Design review of the part built by this model. Coordinates are the model's own, in mm. A direction names the side the tool comes from. Coordinates: 2 decimals unless noted, no trailing zeros. Loops run counter-clockwise (first coordinate to the right, second up) from the corner with the lowest first, then second, coordinate; pieces in that order, holes last.
from build123d import *
from build123d.topology import SkipClean

# Parameters (mm, degrees)
SKETCH1_W           = 60
SKETCH1_H           = 60
BOSS_EXTRUDE1_DEPTH = 3
SKETCH4_W           = 8
SKETCH4_H           = 12
SKETCH4_W_2         = 12
SKETCH4_H_2         = 8
BOSS_EXTRUDE3_DEPTH = 41
SKETCH5_R           = 2
CUT_EXTRUDE2_DEPTH  = 6
SKETCH8_R           = 7.5
CUT_EXTRUDE4_DEPTH  = 6
CUT_EXTRUDE5_DEPTH  = 6
CUT_EXTRUDE6_DEPTH  = 6
SKETCH11_W          = 23.25
SKETCH11_H          = 3
CUT_EXTRUDE7_DEPTH  = 6
SKETCH12_R          = 3
CUT_EXTRUDE8_DEPTH  = 2
SKETCH13_R          = 1.75
CUT_EXTRUDE9_DEPTH  = 1
CHAMFER1_SIZE       = 2
CHAMFER2_SIZE       = 2
CHAMFER3_SIZE       = 2
CUT_EXTRUDE10_DEPTH = 10
FILLET1_R           = 10
CUT_EXTRUDE11_DEPTH = 59.999486357


with BuildPart() as part:
    # Sketch1 → Boss-Extrude1 (new body)
    with BuildSketch(Plane(origin=(0, 0, 0), x_dir=(1, 0, 0), z_dir=(0, 1, 0))):
        Rectangle(SKETCH1_W, SKETCH1_H)
    extrude(amount=BOSS_EXTRUDE1_DEPTH)

    # Sketch4 → Boss-Extrude3 (add)
    with BuildSketch(Plane.XZ):
        with Locations((-26, 0)):
            Rectangle(SKETCH4_W, SKETCH4_H)
        with Locations((0, -26)):
            Rectangle(SKETCH4_W_2, SKETCH4_H_2)
        with Locations((26, 0)):
            Rectangle(SKETCH4_W, SKETCH4_H)
    extrude(amount=BOSS_EXTRUDE3_DEPTH)

    # Sketch5 → Cut-Extrude2 (cut)
    with BuildSketch(Plane.XZ.offset(41)):
        with Locations(Location((0, -26.5, 0), (0, 0, 270))):
            Circle(SKETCH5_R)
        with Locations(Location((-26.5, 0, 0), (0, 0, 270))):
            Circle(SKETCH5_R)
        with Locations(Location((26.5, 0, 0), (0, 0, 270))):
            Circle(SKETCH5_R)
    extrude(amount=-CUT_EXTRUDE2_DEPTH, mode=Mode.SUBTRACT)

    # Sketch8 → Cut-Extrude4 (cut)
    with BuildSketch(Plane(origin=(0, 3, 0), x_dir=(1, 0, 0), z_dir=(0, 1, 0))):
        with Locations(Location((0, 0, 0), (0, 0, 270))):
            Circle(SKETCH8_R)
    extrude(amount=-CUT_EXTRUDE4_DEPTH, mode=Mode.SUBTRACT)

    # Sketch7 → Cut-Extrude5 (cut)
    with BuildSketch(Plane.XZ):
        Polygon((-30, -6), (-6, -30), (-30, -30), align=None)
        Polygon((30, -6), (6, -30), (30, -30), align=None)
    extrude(amount=-CUT_EXTRUDE5_DEPTH, mode=Mode.SUBTRACT)

    # Sketch10 → Cut-Extrude6 (cut)
    with BuildSketch(Plane.XZ):
        Polygon((-9, 30), (-30, 6), (-30, 30), align=None)
        Polygon((9, 30), (30, 6), (30, 30), align=None)
    extrude(amount=-CUT_EXTRUDE6_DEPTH, mode=Mode.SUBTRACT)

    # Sketch11 → Cut-Extrude7 (cut)
    with BuildSketch(Plane.XZ):
        with Locations((0, 28.5)):
            Rectangle(SKETCH11_W, SKETCH11_H)
    extrude(amount=-CUT_EXTRUDE7_DEPTH, mode=Mode.SUBTRACT)

    # Sketch12 → Cut-Extrude8 (cut)
    with BuildSketch(Plane.XZ):
        with Locations(Location((-8, 8, 0), (0, 0, 270))):
            Circle(SKETCH12_R)
        with Locations(Location((8, 8, 0), (0, 0, 270))):
            Circle(SKETCH12_R)
        with Locations(Location((8, -8, 0), (0, 0, 270))):
            Circle(SKETCH12_R)
        with Locations(Location((-8, -8, 0), (0, 0, 270))):
            Circle(SKETCH12_R)
    extrude(amount=-CUT_EXTRUDE8_DEPTH, mode=Mode.SUBTRACT)

    # Sketch13 → Cut-Extrude9 (cut)
    with BuildSketch(Plane(origin=(0, 3, 0), x_dir=(1, 0, 0), z_dir=(0, 1, 0))):
        with Locations(Location((-8, 8, 0), (0, 0, 270))):
            Circle(SKETCH13_R)
        with Locations(Location((8, 8, 0), (0, 0, 270))):
            Circle(SKETCH13_R)
        with Locations(Location((8, -8, 0), (0, 0, 270))):
            Circle(SKETCH13_R)
        with Locations(Location((-8, -8, 0), (0, 0, 270))):
            Circle(SKETCH13_R)
    extrude(amount=-CUT_EXTRUDE9_DEPTH, mode=Mode.SUBTRACT)

    # Chamfer1
    chamfer1_edges = [part.edges().sort_by_distance(p)[0] for p in [
        (30, 3, 0),
        (0, 3, -30),
        (-30, 3, 0),
    ]]
    chamfer(chamfer1_edges, length=CHAMFER1_SIZE)

    # Chamfer2
    chamfer2_edges = [part.edges().sort_by_distance(p)[0] for p in [
        (0, 3, 27),
    ]]
    chamfer(chamfer2_edges, length=CHAMFER2_SIZE)

    # Chamfer3
    chamfer3_edges = [part.edges().sort_by_distance(p)[0] for p in [
        (6, -20.5, -30),
        (-6, -20.5, -30),
        (-30, -20.5, -6),
        (-30, -20.5, 6),
        (30, -20.5, 6),
        (30, -20.5, -6),
    ]]
    chamfer(chamfer3_edges, length=CHAMFER3_SIZE)

    # Sketch14 → Cut-Extrude10 (cut)
    with BuildSketch(Plane.XZ):
        Polygon((-30, -4), (-4, -30), (-6, -30), (-30, -6), align=None)
        Polygon((4, -30), (30, -4), (30, -6), (6, -30), align=None)
    extrude(amount=-CUT_EXTRUDE10_DEPTH, mode=Mode.SUBTRACT)

    # Fillet1
    # the kernel refuses this fillet: 10 mm, written as the material it takes off along each edge
    with BuildSketch(Plane(origin=(-4, 11.355339059, -30), x_dir=(1, 0, 0), z_dir=(0, -1, 0)), Plane(origin=(4, -51.355339059, -30), x_dir=(-1, 0, 0), z_dir=(0, 1, 0)), Plane(origin=(30, 11.355339059, -4), x_dir=(0, 0, 1), z_dir=(0, -1, 0))) as fillet1_piece_1:
        with BuildLine():
            CenterArc((FILLET1_R * 0.414213562373, FILLET1_R), FILLET1_R, 225, 45)
            Line((-FILLET1_R * 0.292893218813, FILLET1_R * 0.292893218813), (0, 0))
            Line((0, 0), (FILLET1_R * 0.414213562373, 0))
        make_face()
    extrude(amount=62.710678119, mode=Mode.SUBTRACT)
    with BuildSketch(Plane(origin=(-30, 0, 4), x_dir=(0, 0, -1), z_dir=(0, -1, 0))) as fillet1_piece_2:
        with BuildLine():
            CenterArc((4, 10), FILLET1_R, 233.130102354, 36.869897646)
            Line((-2, 2), (0, 0))
            Line((0, 0), (4, 0))
        make_face()
    extrude(amount=51, mode=Mode.SUBTRACT)
    with BuildSketch(Plane(origin=(-30, 11.355339059, -4), x_dir=(0, 0, 1), z_dir=(0, -1, 0))) as fillet1_piece_3:
        with BuildLine():
            CenterArc((FILLET1_R * 0.414213562373, -FILLET1_R), FILLET1_R, 90, 45)
            Line((-FILLET1_R * 0.292893218813, -FILLET1_R * 0.292893218813), (0, 0))
            Line((0, 0), (FILLET1_R * 0.414213562373, 0))
        make_face()
    extrude(amount=62.710678119, mode=Mode.SUBTRACT)
    with BuildSketch(Plane(origin=(30, 0, 4), x_dir=(0, 0, -1), z_dir=(0, -1, 0))) as fillet1_piece_4:
        with BuildLine():
            CenterArc((4, -10), FILLET1_R, 90, 36.869897646)
            Line((-2, -2), (0, 0))
            Line((0, 0), (4, 0))
        make_face()
    extrude(amount=51, mode=Mode.SUBTRACT)

    # Sketch16 → Cut-Extrude11 (cut, through all)
    with SkipClean():  # the faces are left unmerged after this step: merging them gives an invalid solid
        with BuildSketch(Plane.XZ):
            with BuildLine():
                Line((-28, 6), (-9.625, 27))
                Line((-9.625, 27), (-11.625, 27))
                Line((-11.625, 27), (-30, 6))
                Line((-30, 6), (-30, 0.142135624))
                ThreePointArc((-30, 0.142135624), (-29.999936866, 0.106601493), (-29.999747465, 0.071067812))
                ThreePointArc((-29.999747465, 0.071067812), (-29.475536208, 3.195968331), (-28, 6))
            make_face()
            with BuildLine():
                Line((28, 6), (9.625, 27))
                Line((9.625, 27), (11.625, 27))
                Line((11.625, 27), (30, 6))
                Line((30, 6), (30, 0.142135624))
                ThreePointArc((30, 0.142135624), (29.999936866, 0.106601493), (29.999747465, 0.071067812))
                ThreePointArc((29.999747465, 0.071067812), (29.475536208, 3.195968331), (28, 6))
            make_face()
        extrude(amount=-CUT_EXTRUDE11_DEPTH, mode=Mode.SUBTRACT)


solid = part.part
Q1. Machinability: for faces 4 (the flat face through (-6, -20, -25)), 5 (the cylindrical face through (24.548, -38.042, 0.434)), 6 (the flat face through (22, -20, 0)), which of the approach directions +Z, -Z, +X, -X, +Y, -Y give a long, thin tool a straight path to every point of the face, cutting with its end or side? Answer none if there is none.
Q2. For line 1 (X direction, y = 2.6, z = -8); line 2 (X direction, y = 0.5, z = -8); line 3 (Y direction, x = -21, z = 13), list the stretches that pass through material, from the lowest coordinate up.
Q3. Take a section at A-A, the plane y = -37.5. Write out the cut boundary in (x, z).
Q4. Take a section at C-C, the plane z = 4. Write out the cut boundary in (x, y).
Q5. Take a section at D-D, the plane x = 25.5. Write out the cut boundary in (y, z), then the cut area to 3 significant figures.
Q6. Clearance check with flat-ended pins moving along their axes: pin 1 Ø3 at (y, z) = (-19.5, -23.5) entering from -X; pin 2 Ø5 at (x, z) = (8.5, -8.5) entering from -Y; pin 3 Ø5 at (x, y) = (-3, -3.5) entering from -Z. State where each tip first meets the part, or that it passes through.
Q7. The part is to be moulded in two halves that separate along Z. For faces 1 (the flat face through (29, 2, 0)), 2 (the cylindrical face through (2.999, -19.308, -29.494)), 3 (the flat face through (-8, 2, 6)), say which applies: pulls with the +Z half, pulls with the -Z half, needs draft (parallel to the pull), parting line crosses it, or undercut.
Q8. Take a section at B-B, the plane x = 4. Write out the cut boundary in (y, z), then the cut area to 3 significant figures.
Entries:
1. face 4: +Z, -Z, -X, -Y
1. face 5: -Y
1. face 6: +Z, -Z, -Y
2. line 1: x = -26 to -9.75, -6.25 to 6.25, 9.75 to 26
2. line 2: x = -26 to -11, -5 to 5, 11 to 26
2. line 3: y = 0 to 3
3. outline: (-30, 0.07) arc R10 ccw to (-27.89, -6) - (-22, -6) - (-22, 6) - (-28, 6) arc R10 ccw to start; (-6, -27.89) arc R10 ccw to (0, -30) arc R10 ccw to (6, -27.89) - (6, -22) - (-6, -22) - close; (22, -6) - (27.89, -6) arc R10 ccw to (30, 0.07) arc R10 ccw to (28, 6) - (22, 6) - close; hole circle Ø4 at (-26.5, 0); hole circle Ø4 at (0, -26.5); hole circle Ø4 at (26.5, 0)
4. outline: (-29.17, -41) - (-22, -41) - (-22, 0) - (-6.34, 0) - (-6.34, 3) - (-28, 3) - (-29.17, 1.83) - close; (6.34, 0) - (22, 0) - (22, -41) - (29.17, -41) - (29.17, 1.83) - (28, 3) - (6.34, 3) - close
5. outline: (-41, -6) - (0, -6) - (0, -8.5) - (3, -8.5) - (3, 8.86) - (0, 8.86) - (0, 6) - (-41, 6) - (-41, 1.73) - (-35, 1.73) - (-35, -1.73) - (-41, -1.73) - close
5. area: 523 mm2
6. pin 1: stops at x = -6
6. pin 2: stops at y = 0
6. pin 3: stops at z = -29.98
7. face 1: needs draft
7. face 2: pulls with the -Z half
7. face 3: undercut
8. outline: (-41, -29.1) - (1.9, -29.1) - (3, -28) - (3, -6.34) - (0, -6.34) - (0, -22) - (-41, -22) - close; (0, 6.34) - (3, 6.34) - (3, 25) - (1, 27) - (0, 27) - close
8. area: 419 mm2
